Verification items for the finished model (mm, model axes). Face numbers are marked on the shaded views. A direction names the side the tool comes from. Give positions to 0.01 mm unless a question says otherwise; leave off trailing zeros. Order: outer loops, then holes, each group sorted by start corner. A loop starts at its lowest first (then second) coordinate and runs counter-clockwise, first axis right, second up. Notation, with made-up numbers: (71, -40) - (91, -40) arc R13 ccw to (91, -34) - close; hole circle Ø5 at (10, 71). An arc over 180 degrees is marked (long way). Answer as a JSON object with one key per item and string values.
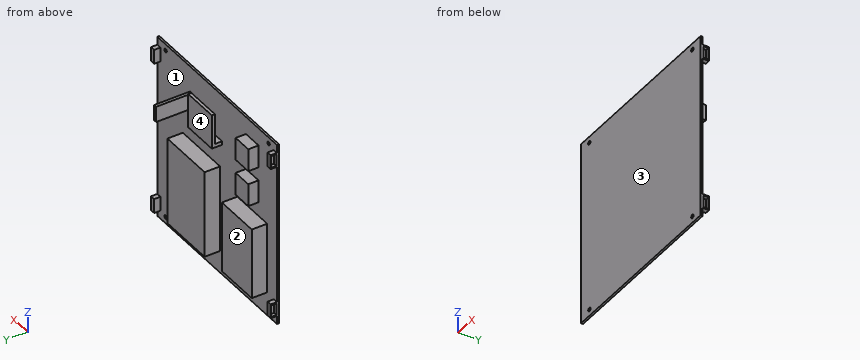
```python
from build123d import *

# Parameters (mm, degrees)
SKETCH_1_W                                 = 180
SKETCH_1_H                                 = 180
EXTRUDE_1_DEPTH                            = 2
SKETCH_2_W                                 = 4.7
SKETCH_2_H                                 = 14
EXTRUDE_2_DEPTH                            = 6.05
SKETCH_3_W                                 = 11.570247934
SKETCH_3_H                                 = 5
CUT_EXTRUDE_1_DEPTH                        = 3.5
MIRROR_1_AT_THE_SECOND_PLANE_COPY_1_SKET_W = 11.570247934
MIRROR_1_AT_THE_SECOND_PLANE_COPY_1_SKET_H = 5
MIRROR_1_AT_THE_SECOND_PLANE_COPY_1_DEPTH  = 3.5
SKETCH_4_W                                 = 45
SKETCH_4_H                                 = 69
EXTRUDE_3_DEPTH                            = 15
SKETCH_5_W                                 = 19
SKETCH_5_H                                 = 22
EXTRUDE_4_DEPTH                            = 10
SKETCH_6_W                                 = 56
SKETCH_6_H                                 = 85
EXTRUDE_5_DEPTH                            = 15
SKETCH_7_W                                 = 35.4
SKETCH_7_H                                 = 33.5
EXTRUDE_6_DEPTH                            = 10
SKETCH_8_W                                 = 35.4
SKETCH_8_H                                 = 7
CUT_EXTRUDE_6_DEPTH                        = 30
SKETCH_9_W                                 = 3
SKETCH_9_H                                 = 15.3
EXTRUDE_7_DEPTH                            = 35
SKETCH_10_R                                = 1.8
CUT_EXTRUDE_7_DEPTH                        = 10
MIRROR_3_AT_THE_SECOND_PLANE_COPY_1_SKET_R = 1.8
MIRROR_3_AT_THE_SECOND_PLANE_COPY_1_DEPTH  = 10


with BuildPart() as part:
    # 草图1 → 凸台-拉伸1 (new body)
    with BuildSketch(Plane(origin=(0, 0, 0), x_dir=(1, 0, 0), z_dir=(0, 1, 0))):
        Rectangle(SKETCH_1_W, SKETCH_1_H)
    extrude(amount=EXTRUDE_1_DEPTH)

    # 草图2 → 凸台-拉伸2 (add)
    with BuildSketch(Plane(origin=(0, 2, 0), x_dir=(1, 0, 0), z_dir=(0, 1, 0))):
        with Locations((-87.65, 75)):
            Rectangle(SKETCH_2_W, SKETCH_2_H)
        with Locations((-87.65, -75)):
            Rectangle(SKETCH_2_W, SKETCH_2_H)
        with Locations((87.65, -75)):
            Rectangle(SKETCH_2_W, SKETCH_2_H)
        with Locations((87.65, 75)):
            Rectangle(SKETCH_2_W, SKETCH_2_H)
    extrude(amount=EXTRUDE_2_DEPTH)

    # 草图3 → 切除-拉伸1 (cut)
    with BuildSketch(Plane.ZY.offset(90)):
        with Locations((-75, 5.025)):
            Rectangle(SKETCH_3_W, SKETCH_3_H)
    cut_extrude_1 = extrude(amount=-CUT_EXTRUDE_1_DEPTH, mode=Mode.SUBTRACT)

    # 镜向1: 切除-拉伸1 across plane
    add(cut_extrude_1.mirror(Plane(origin=(0, 0, 0), x_dir=(0, 0, 1), z_dir=(1, 0, 0))), mode=Mode.SUBTRACT)

    # 镜向1 at the second plane: 切除-拉伸1 across plane
    add(cut_extrude_1.mirror(Plane.XY), mode=Mode.SUBTRACT)

    # 镜向1 at the second plane copy 1 sket → 镜向1 at the second plane copy 1 (cut)
    with BuildSketch(Plane(origin=(90, 0, 0), x_dir=(0, 0, -1), z_dir=(1, 0, 0))):
        with Locations((-75, 5.025)):
            Rectangle(MIRROR_1_AT_THE_SECOND_PLANE_COPY_1_SKET_W, MIRROR_1_AT_THE_SECOND_PLANE_COPY_1_SKET_H)
    extrude(amount=-MIRROR_1_AT_THE_SECOND_PLANE_COPY_1_DEPTH, mode=Mode.SUBTRACT)

    # 草图4 → 凸台-拉伸3 (add)
    with BuildSketch(Plane(origin=(0, 2, 0), x_dir=(1, 0, 0), z_dir=(0, 1, 0))):
        with Locations((-52.915832737, 32.492177997)):
            Rectangle(SKETCH_4_W, SKETCH_4_H)
    extrude(amount=EXTRUDE_3_DEPTH)

    # 草图5 → 凸台-拉伸4 (add)
    with BuildSketch(Plane(origin=(0, 2, 0), x_dir=(1, 0, 0), z_dir=(0, 1, 0))):
        with Locations((-52.915832737, -26.729978553)):
            Rectangle(SKETCH_5_W, SKETCH_5_H)
        with Locations((-52.915832737, -61.854870093)):
            Rectangle(SKETCH_5_W, SKETCH_5_H)
    extrude(amount=EXTRUDE_4_DEPTH)

    # 草图6 → 凸台-拉伸5 (add)
    with BuildSketch(Plane(origin=(0, 2, 0), x_dir=(1, 0, 0), z_dir=(0, 1, 0))):
        with Locations((23.523310823, 25.733573793)):
            Rectangle(SKETCH_6_W, SKETCH_6_H)
    extrude(amount=EXTRUDE_5_DEPTH)

    # 草图7 → 凸台-拉伸6 (add)
    with BuildSketch(Plane(origin=(0, 2, 0), x_dir=(1, 0, 0), z_dir=(0, 1, 0))):
        with Locations((10.21182737, -57.09339848)):
            Rectangle(SKETCH_7_W, SKETCH_7_H)
    extrude(amount=EXTRUDE_6_DEPTH)

    # 草图8 → 切除-拉伸6 (cut)
    with BuildSketch(Plane.XY.offset(73.84339848)):
        with Locations((10.21182737, 5.5)):
            Rectangle(SKETCH_8_W, SKETCH_8_H)
    extrude(amount=-CUT_EXTRUDE_6_DEPTH, mode=Mode.SUBTRACT)

    # 草图9 → 凸台-拉伸7 (add)
    with BuildSketch(Plane(origin=(0, 2, 0), x_dir=(1, 0, 0), z_dir=(0, 1, 0))):
        with Locations((38.990613596, -57.325485465)):
            Rectangle(SKETCH_9_W, SKETCH_9_H)
    extrude(amount=EXTRUDE_7_DEPTH)

    # 草图10 → 切除-拉伸7 (cut)
    with BuildSketch(Plane(origin=(0, 2, 0), x_dir=(1, 0, 0), z_dir=(0, 1, 0))):
        with Locations(Location((77.5, 83.802246308, 0), (0, 0, 270))):
            Circle(SKETCH_10_R)
    cut_extrude_7 = extrude(amount=-CUT_EXTRUDE_7_DEPTH, mode=Mode.SUBTRACT)

    # 镜向3: 切除-拉伸7 across plane
    add(cut_extrude_7.mirror(Plane(origin=(0, 0, 0), x_dir=(0, 0, 1), z_dir=(1, 0, 0))), mode=Mode.SUBTRACT)

    # 镜向3 at the second plane: 切除-拉伸7 across plane
    add(cut_extrude_7.mirror(Plane.XY), mode=Mode.SUBTRACT)

    # 镜向3 at the second plane copy 1 sket → 镜向3 at the second plane copy 1 (cut)
    with BuildSketch(Plane(origin=(0, 2, 0), x_dir=(-1, 0, 0), z_dir=(0, 1, 0))):
        with Locations(Location((77.5, 83.802246308, 0), (0, 0, 270))):
            Circle(MIRROR_3_AT_THE_SECOND_PLANE_COPY_1_SKET_R)
    extrude(amount=-MIRROR_3_AT_THE_SECOND_PLANE_COPY_1_DEPTH, mode=Mode.SUBTRACT)


solid = part.part
```
(1) Section check C-C (x = -71.5). Record the cut outline in (y, z).
Computed values:
{"outline": "(0, -90) - (2, -90) - (2, -66.99) - (17, -66.99) - (17, 2.01) - (2, 2.01) - (2, 90) - (0, 90) - close"}
(2) Access from +Z, -Z, +X, -X, +Y, -Y to the whole of each face (thin tool, end or side, straight path). Record for the marked faces 3 and 4.
Computed values:
{"face 3": "+Z, -Z, +X, -X, -Y", "face 4": "+Z, -X, +Y"}
(3) Section check A-A (z = 53). Record the cut outline in (x, y).
Computed values:
{"outline": "(-90, 0) - (90, 0) - (90, 2) - (40.49, 2) - (40.49, 37) - (37.49, 37) - (37.49, 2) - (-43.42, 2) - (-43.42, 12) - (-62.42, 12) - (-62.42, 2) - (-90, 2) - close; (-7.49, 9) - (27.91, 9) - (27.91, 12) - (-7.49, 12) - close"}
(4) Section check D-D (y = 20.5). Record the cut outline in (x, z).
Computed values:
{"outline": "(37.49, 49.68) - (40.49, 49.68) - (40.49, 64.98) - (37.49, 64.98) - close"}
(5) Gauge pin test, flat ends, axial feed: pin 1 Ø1 at (x, y) = (88, 5.5) entering from +Z; pin 2 Ø4 at (y, z) = (4, 75) entering from -X; pin 3 Ø5 at (x, z) = (-12, -42.5) entering from +Y; pin 4 Ø2.5 at (x, y) = (-87.5, 4) entering from -Z. Record the tip position at first contact, or that the pin passes through.
Computed values:
{"pin 1": "stops at z = 82", "pin 2": "stops at x = -90", "pin 3": "stops at y = 2", "pin 4": "stops at z = -82"}
(6) Release check for a two-part mould opening along X. For the marked faces 1 and 2 record: pulls with the +X half, pulls with the -X half, needs draft (parallel to the pull), parting line crosses it, or undercut.
Computed values:
{"face 1": "undercut", "face 2": "needs draft"}
(7) Material ranges on line 1 along Z through (x, y) = (-77.5, 1.2); line 2 along Z through (x, y) = (77, 1); line 3 along Y through (x, z) = (-34, 47), recorded low to high. Write a range as [from, to].
Computed values:
{"line 1": "z = [-90, -85.6], [-82, 82], [85.6, 90]", "line 2": "z = [-90, -85.53], [-82.07, 82.07], [85.53, 90]", "line 3": "y = [0, 2]"}
(8) Section check B-B (z = -33.5). Record the cut outline in (x, y), then the cut area to 4 significant figures.
Computed values:
{"outline": "(-90, 0) - (90, 0) - (90, 2) - (51.52, 2) - (51.52, 17) - (-4.48, 17) - (-4.48, 2) - (-30.42, 2) - (-30.42, 17) - (-75.42, 17) - (-75.42, 2) - (-90, 2) - close", "area": "1,875 mm²"}
